Here's how the part is built. I have some questions about the finished solid (model axes, mm). A direction names the side the tool comes from. Coordinates: 2 decimals unless noted, no trailing zeros. Write each loop counter-clockwise with the first axis right and the second up, starting at its lowest first coordinate (ties: lowest second). Pieces come first, ordered by that corner, then holes. Notation, with made-up numbers: (-2, 14.5) -> (3, 14.5) arc R22 cw to (3, 33.5) -> close; hole circle Ø6 at (-30.75, 32.5). An arc over 180 degrees is marked (long way). Answer in a Markdown table with one row per item. Add a question column.
from build123d import *

# Parameters (mm, degrees)
F1_DEPTH = 2080
F2_W     = 39.969242
F2_H     = 51.200114
F2_H_2   = 66.946672
F2_W_2   = 34.220117
F2_H_3   = 62.673524
F3_DEPTH = 25
F4_W     = 37.147605
F4_H     = 21.549247
F4_H_2   = 14.081187
F4_W_2   = 32.29431
F4_H_3   = 23.482673
F4_H_4   = 16.907938
F5_DEPTH = 25


with BuildPart() as f1:
    # F0 (on Right) → F1 (new body)
    with BuildSketch(Plane.YZ):
        with BuildLine():
            Line((-325, 0), (-6, 0))
            ThreePointArc((-6, 0), (-1.757359, 1.757359), (0, 6))
            Line((0, 6), (0, 12))
            ThreePointArc((0, 12), (-1.757359, 16.242641), (-6, 18))
            Line((-6, 18), (-325, 18))
            ThreePointArc((-325, 18), (-350.844186, 16.306083), (-376.246171, 11.253314))
            Line((-376.246171, 11.253314), (-418.746907, -0.134724))
            ThreePointArc((-418.746907, -0.134724), (-422.390145, -2.930279), (-422.989548, -7.483194))
            Line((-422.989548, -7.483194), (-421.436634, -13.278749))
            ThreePointArc((-421.436634, -13.278749), (-418.641079, -16.921987), (-414.088164, -17.521389))
            Line((-414.088164, -17.521389), (-371.587428, -6.133351))
            ThreePointArc((-371.587428, -6.133351), (-348.494715, -1.539925), (-325, 0))
        make_face()
    extrude(amount=F1_DEPTH)

    # F2 (on face) → F3 (cut)
    with BuildSketch(Plane.XY.offset(18)):
        with Locations((2081.984621, -10.399943)):
            Rectangle(F2_W, F2_H)
        with Locations((2081.984621, -328.473336)):
            Rectangle(F2_W, F2_H_2)
        with Locations((0.889942, -328.473336)):
            Rectangle(F2_W_2, F2_H_2)
        with Locations((0.889942, -4.663238)):
            Rectangle(F2_W_2, F2_H_3)
    extrude(amount=-F3_DEPTH, mode=Mode.SUBTRACT)

    # F4 (on face) → F5 (cut)
    with BuildSketch(Plane(origin=(0, -28.017043, 104.561027), x_dir=(1, 0, 0), z_dir=(0, -0.258819, 0.965926))):
        with Locations((-0.573802, -349.738698)):
            Rectangle(F4_W, F4_H)
        with Locations((-0.573802, -411.553915)):
            Rectangle(F4_W, F4_H_2)
        with Locations((2078.147155, -348.771985)):
            Rectangle(F4_W_2, F4_H_3)
        with Locations((2078.147155, -412.967291)):
            Rectangle(F4_W_2, F4_H_4)
    extrude(amount=-F5_DEPTH, mode=Mode.SUBTRACT)


solid = f1.part
Q1. Imagine slicing it at A-A on x = 743. Please give me the cut outline in (y, z), plus the area to 3 significant figures.
Q2. Imagine slicing it at B-B on y = -72.5. Please give me the cut outline in (x, z).
Q3. I need wall thicknesses on line 1 (Z direction, x = 1277, y = -158); line 2 (X direction, y = -30, z = 7); line 3 (Z direction, x = 84, y = -356). Which ranges of each line are inside material? Lowest first, please. Write a range as [from, to].
Q4. For faces 1 (the flat face through (1025, -168, 0)), 2 (the flat face through (1025.44, -397.2, 5.64)), which set-ups out of +Z, -Z, +X, -X, +Y, -Y let a thin tool reach every point of the face, with its end or its side?
Q5. Imagine slicing it at C-C on y = -350. Please give me the cut outline in (x, z), plus the area to 3 significant figures.
Q6. I'm going to push flat-ended pins straight in: P1, Ø2, axis at x = 1212, y = -362.5, coming from the +Z side; P2, Ø14.5, axis at y = -23.5, z = 5, coming from the +X side; P3, Ø5.5, axis at x = 2067, z = 6, coming from the +Y side. Where does each tip first touch, or does it pass through?
Result sheet:
| question | item | result |
|---|---|---|
| 1 | outline | (-422.99, -7.48) -> (-421.44, -13.28) arc R6 ccw to (-414.09, -17.52) -> (-371.59, -6.13) arc R180 cw to (-325, 0) -> (-6, 0) arc R6 ccw to (0, 6) -> (0, 12) arc R6 ccw to (-6, 18) -> (-325, 18) arc R198 ccw to (-376.25, 11.25) -> (-418.75, -0.13) arc R6 ccw to start |
| 1 | area | 7,610 mm^2 |
| 2 | outline | (0, 0) -> (2080, 0) -> (2080, 18) -> (0, 18) -> close |
| 3 | line 1 | z = [0, 18] |
| 3 | line 2 | x = [18, 2062] |
| 3 | line 3 | z = [-2.69, 15.56] |
| 4 | face 1 | -Z, +X, -X, +Y |
| 4 | face 2 | +Z, +X, -X, -Y |
| 5 | outline | (18, -1.74) -> (2062, -1.74) -> (2062, 16.42) -> (18, 16.42) -> close |
| 5 | area | 37,100 mm^2 |
| 6 | P1 | stops at z = 14.61 |
| 6 | P2 | stops at x = 2062 |
| 6 | P3 | stops at y = -36 |
